Read the model definition and answer for the solid it produces. Units are mm, in the model's axes. Face numbers are marked on the shaded views. A direction names the side the tool comes from. Coordinates: 2 decimals unless noted, no trailing zeros. Loops run counter-clockwise (first coordinate to the right, second up) from the corner with the lowest first, then second, coordinate; pieces in that order, holes last. Notation, with made-up numbers: (-12, 81.25) - (40, 81.25) arc R15 cw to (40, 109.25) - close; hole circle Ø9 at (88, 24.25). An arc over 180 degrees is marked (long way). One line per question, with ' | ' between items. Start each with the question number.
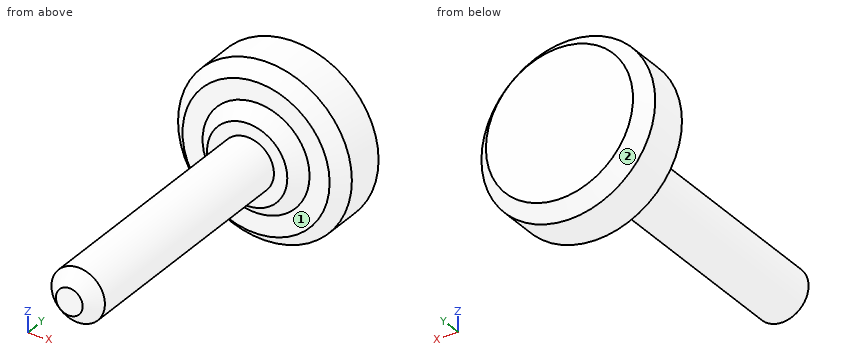
Autodesk Inventor part; units mm, degrees
ref_plane "YZ Plane" through (0, 0, 0) normal (1, 0, 0) x (0, 1, 0)
ref_plane "XZ Plane" through (0, 0, 0) normal (0, 1, 0) x (-1, 0, 0)
ref_plane "XY Plane" through (0, 0, 0) normal (0, 0, 1) x (1, 0, 0)
sketch "Body Cross Section" plane through (0, 0, 0) normal (0, 1, 0) x (-1, 0, 0)
  circle A0 centre (0, 0) radius 4
  dimension "d0" = 8
extrude "Body" add sketch "Body Cross Section" against normal blind 40
sketch "Base Cross Section" plane through (0, 0, 0) normal (0, 1, 0) x (1, 0, 0)
  circle A0 centre (0, 0) radius 8
  dimension "d3" = 16
extrude "Base" add sketch "Base Cross Section" along normal blind 2
sketch "Head Cross Section" plane through (0, 2, 0) normal (0, 1, 0) x (1, 0, 0)
  circle A0 centre (0, 0) radius 13
  dimension "d6" = 26
extrude "Head" add sketch "Head Cross Section" along normal blind 10
thread "Thread"
chamfer "Body Chamfer" distance 2 angle 45 1 edges at (4, -40, 0)
chamfer "Head Chamfer" distance 2 angle 45 3 edges at (-13, 12, 0) (-13, 2, 0) (-8, 0, 0)
properties part number "P0480.080-040-A4" material "Stainless Steel AISI 317"
1) Find the intervals of material crossed by line 1 along Y through (x, z) = (7, -8); line 2 along Y through (x, z) = (2.5, 11.5); line 3 along X through (y, z) = (7, 11.5), in increasing order. Write a range as from..to.
2) The part is cut by section C-C on y = -23. Write down the section's boundary in (x, z), and give its area (3 significant figures).
3) Which of the six approach directions +Z, -Z, +X, -X, +Y, -Y give full straight-line access (tool end or side, diameter ignored) to the marked faces 1 and 2?
4) Given pin 1 Ø2 at (x, z) = (-5.5, 0.5) entering from -Y; pin 2 Ø3 at (x, z) = (-0.5, -10) entering from -Y; pin 3 Ø2 at (y, z) = (-33.5, -2) entering from -X, each flat-ended and moving along its own axis, determine where each tip first touches the part or whether it passes through.
Answer below:
1) line 1: 2..12 | line 2: 2.77..11.23 | line 3: -6.06..6.06
2) outline: circle Ø8 at (0, 0) | area: 50.3 mm2
3) face 1: -Y | face 2: +Y
4) pin 1: y = 0 | pin 2: y = 2 | pin 3: x = -3.87
